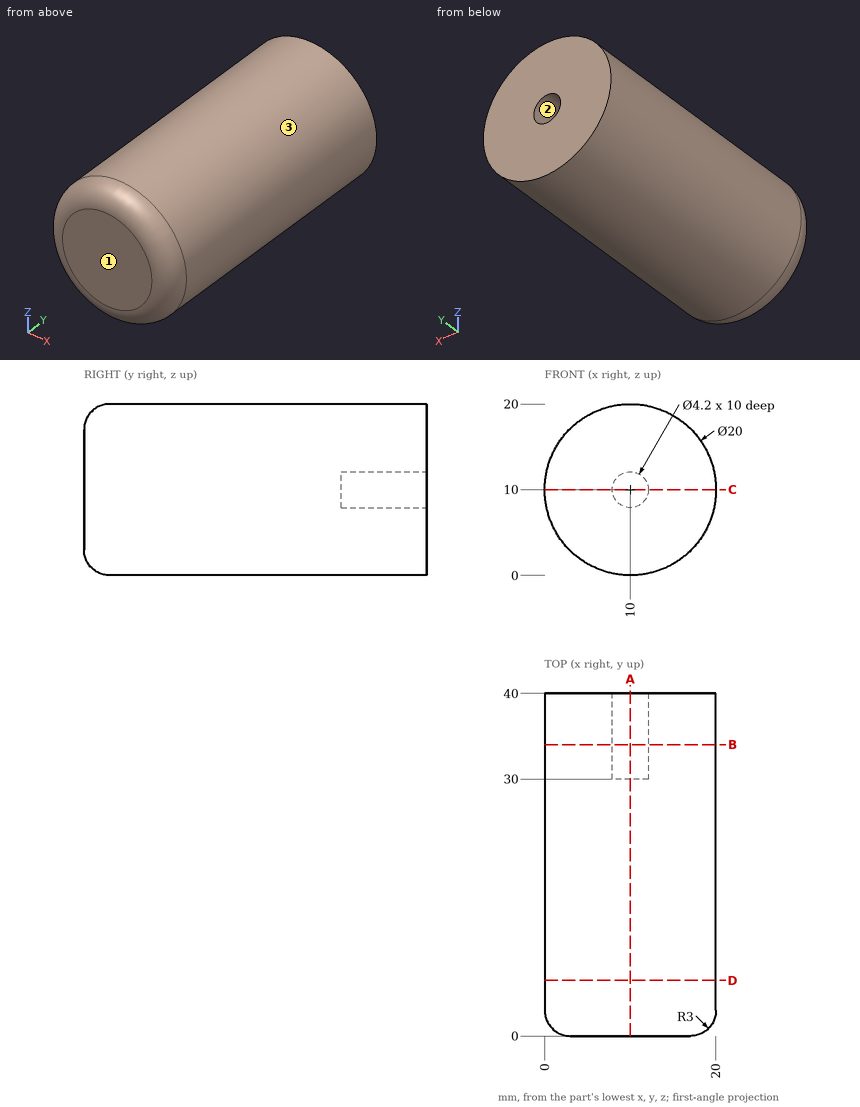
Job drawing, mm, ordinate dimensions from the low corner. One solid piece. Round coordinates to 2 decimals unless told otherwise and drop trailing zeros. Loops run counter-clockwise (first coordinate to the right, second up) from the corner with the lowest first, then second, coordinate; pieces in that order, holes last. Notation, with made-up numbers: (33, 4.5) -> (45, 4.5) arc R21 cw to (45, 36.5) -> close; hole circle Ø2 at (78, 34.25). An arc over 180 degrees is marked (long way). Use CSV: the item, a comma, the result in double quotes. Start each with the question number.
Q1. Saw through at C-C on z = 10. Give the cut face in (x, y), and give its area (3 significant figures).
Q2. Flat gauge pins, fed straight in: pin 1 Ø8 at (y, z) = (9, 16.5) entering from +X; pin 2 Ø2 at (x, z) = (10, 9.5) entering from +Y; pin 3 Ø3 at (y, z) = (22.5, 4) entering from +X. Where does each tip first touch, or does it go through?
Q3. Saw through at A-A on x = 10. Give the cut face in (y, z).
Q4. Saw through at D-D on y = 6.5. Give the cut face in (x, z), and give its area (3 significant figures).
Q5. Saw through at B-B on y = 34. Give the cut face in (x, z).
Q6. Drill centre lines: L1, parallel to Z at x = 10, y = 32.5; L2, parallel to X at y = 30.5, z = 11.25. Where is each one in solid material? Low to high.
Q7. Mould opens along X. For the marked faces 1, 2 and 3 say: +X half, -X half, draft (parallel to the pull), parting line (faces both ways), or undercut.
Solutions:
1,outline,"(0, 3) arc R3 ccw to (3, 0) -> (17, 0) arc R3 ccw to (20, 3) -> (20, 40) -> (12.1, 40) -> (12.1, 30) -> (7.9, 30) -> (7.9, 40) -> (0, 40) -> close"
1,area,"754 mm^2"
2,pin 1,"stops at x = 19.68"
2,pin 2,"stops at y = 30"
2,pin 3,"stops at x = 18.93"
3,outline,"(0, 3) arc R3 ccw to (3, 0) -> (40, 0) -> (40, 7.9) -> (30, 7.9) -> (30, 12.1) -> (40, 12.1) -> (40, 20) -> (3, 20) arc R3 ccw to (0, 17) -> close"
4,outline,"circle Ø20 at (10, 10)"
4,area,"314 mm^2"
5,outline,"circle Ø20 at (10, 10); hole circle Ø4.2 at (10, 10)"
6,L1,"z = 0 to 7.9, 12.1 to 20"
6,L2,"x = 0.08 to 8.31, 11.69 to 19.92"
7,face 1,"draft"
7,face 2,"undercut"
7,face 3,"parting line"
